```python
from build123d import *

# Parameters (mm, degrees)
SKETCH1_W                = 259.08
SKETCH1_H                = 298.45
BOSS_EXTRUDE3_DEPTH      = 14.732
SKETCH2_W                = 259.08
SKETCH2_H                = 298.45
BOSS_EXTRUDE4_DEPTH      = 22.098
SKETCH4_OUTSIDE_W        = 379.836
SKETCH4_OUTSIDE_H        = 118.216
CUT_EXTRUDE2_DEPTH       = 259.08
SKETCH6_OUTSIDE_W        = 340.466
SKETCH6_OUTSIDE_H        = 118.216
CUT_EXTRUDE4_DEPTH       = 298.45
BOSS_EXTRUDE6_DEPTH      = 101.6
BOSS_EXTRUDE6_DEPTH_BACK = 101.6
SKETCH8_W                = 88.392
SKETCH8_H                = 7.62
CUT_EXTRUDE5_DEPTH       = 127
CUT_EXTRUDE7_DEPTH       = 50.8
CUT_EXTRUDE7_DEPTH_BACK  = 50.8
SKETCH15_W               = 25.4
SKETCH15_H               = 6.576785714
CUT_EXTRUDE8_DEPTH       = 53.086
SKETCH16_W               = 25.4
SKETCH16_H               = 6.576785714
CUT_EXTRUDE9_DEPTH       = 53.086
SKETCH17_R               = 5.08
CUT_EXTRUDE10_DEPTH      = 8.62
SKETCH18_R               = 2.54
CUT_EXTRUDE11_DEPTH      = 260.08
SKETCH19_R               = 5.08
CUT_EXTRUDE12_DEPTH      = 8.62
SKETCH21_R               = 5.08
CUT_EXTRUDE13_DEPTH      = 8.62


with BuildPart() as part:
    # Sketch1 → Boss-Extrude3 (new body)
    with BuildSketch(Plane(origin=(0, 0, 0), x_dir=(1, 0, 0), z_dir=(0, 1, 0))):
        Rectangle(SKETCH1_W, SKETCH1_H)
    extrude(amount=BOSS_EXTRUDE3_DEPTH)

    # Sketch2 → Boss-Extrude4 (add)
    with BuildSketch(Plane.XZ):
        Rectangle(SKETCH2_W, SKETCH2_H)
    extrude(amount=BOSS_EXTRUDE4_DEPTH)

    # Sketch4 outside → Cut-Extrude2 (cut)
    with BuildSketch(Plane(origin=(129.54, 0, 0), x_dir=(0, 0, -1), z_dir=(1, 0, 0))):
        with Locations((0, -3.683)):
            Rectangle(SKETCH4_OUTSIDE_W, SKETCH4_OUTSIDE_H)
        Polygon((0, -22.098), (-149.225, 0), (-149.225, 14.732), (149.225, 14.732), (149.225, 0), align=None, mode=Mode.SUBTRACT)
    extrude(amount=-CUT_EXTRUDE2_DEPTH, mode=Mode.SUBTRACT)

    # Sketch6 outside → Cut-Extrude4 (cut)
    with BuildSketch(Plane.XY.offset(149.225)):
        with Locations((0, -3.683)):
            Rectangle(SKETCH6_OUTSIDE_W, SKETCH6_OUTSIDE_H)
        Polygon((-44.196, -22.098), (44.196, -22.098), (129.54, 0), (129.54, 14.732), (-129.54, 14.732), (-129.54, 0), align=None, mode=Mode.SUBTRACT)
    extrude(amount=-CUT_EXTRUDE4_DEPTH, mode=Mode.SUBTRACT)


with BuildPart() as body_2:
    # Sketch7 → Boss-Extrude6 (new body, two sides)
    with BuildSketch(Plane.XY) as boss_extrude6_sk:
        Polygon((44.196, -27.178), (129.54, -5.08), (129.54, -34.798), (-129.54, -34.798), (-129.54, -5.08), (-44.196, -27.178), align=None)
    extrude(amount=BOSS_EXTRUDE6_DEPTH)
    extrude(boss_extrude6_sk.sketch, amount=-BOSS_EXTRUDE6_DEPTH_BACK)

    # Sketch8 → Cut-Extrude5 (cut)
    with BuildSketch(Plane.XY.offset(101.6)):
        with Locations((0, -30.988)):
            Rectangle(SKETCH8_W, SKETCH8_H)
    extrude(amount=-CUT_EXTRUDE5_DEPTH, mode=Mode.SUBTRACT)

    # Sketch10 → Cut-Extrude7 (cut, two sides)
    with BuildSketch(Plane.XY) as cut_extrude7_sk:
        Polygon((-44.196, -27.178), (-120.396, -7.447642857), (-120.396, -34.798), (-44.196, -34.798), align=None)
        Polygon((120.396, -7.447642857), (44.196, -27.178), (44.196, -34.798), (120.396, -34.798), align=None)
    extrude(amount=CUT_EXTRUDE7_DEPTH, mode=Mode.SUBTRACT)
    extrude(cut_extrude7_sk.sketch, amount=-CUT_EXTRUDE7_DEPTH_BACK, mode=Mode.SUBTRACT)

    # Sketch15 → Cut-Extrude8 (cut)
    with BuildSketch(Plane.XY.offset(101.6)):
        with Locations((56.896, -23.889607143)):
            Rectangle(SKETCH15_W, SKETCH15_H)
    extrude(amount=-CUT_EXTRUDE8_DEPTH, mode=Mode.SUBTRACT)

    # Sketch16 → Cut-Extrude9 (cut)
    with BuildSketch(Plane.XY.offset(101.6)):
        with Locations((-56.896, -23.889607143)):
            Rectangle(SKETCH16_W, SKETCH16_H)
    extrude(amount=-CUT_EXTRUDE9_DEPTH, mode=Mode.SUBTRACT)

    # Sketch17 → Cut-Extrude10 (cut, through all)
    with BuildSketch(Plane(origin=(0, -27.178, 0), x_dir=(1, 0, 0), z_dir=(0, 1, 0))):
        with Locations((-31.496, 88.9)):
            Circle(SKETCH17_R)
        with Locations((31.496, 88.9)):
            Circle(SKETCH17_R)
    extrude(amount=-CUT_EXTRUDE10_DEPTH, mode=Mode.SUBTRACT)

    # Sketch18 → Cut-Extrude11 (cut, through all)
    with BuildSketch(Plane.ZY.offset(129.54)):
        with Locations((38.1, -19.939)):
            Circle(SKETCH18_R)
        with Locations((-38.1, -19.939)):
            Circle(SKETCH18_R)
    extrude(amount=-CUT_EXTRUDE11_DEPTH, mode=Mode.SUBTRACT)

    # Sketch19 → Cut-Extrude12 (cut, through all)
    with BuildSketch(Plane(origin=(0, -27.178, 0), x_dir=(1, 0, 0), z_dir=(0, 1, 0))):
        with Locations((-56.896, -76.2)):
            Circle(SKETCH19_R)
    extrude(amount=-CUT_EXTRUDE12_DEPTH, mode=Mode.SUBTRACT)

    # Sketch21 → Cut-Extrude13 (cut, through all)
    with BuildSketch(Plane(origin=(0, -27.178, 0), x_dir=(1, 0, 0), z_dir=(0, 1, 0))):
        with Locations((56.896, -76.2)):
            Circle(SKETCH21_R)
    extrude(amount=-CUT_EXTRUDE13_DEPTH, mode=Mode.SUBTRACT)


solid = body_2.part
```
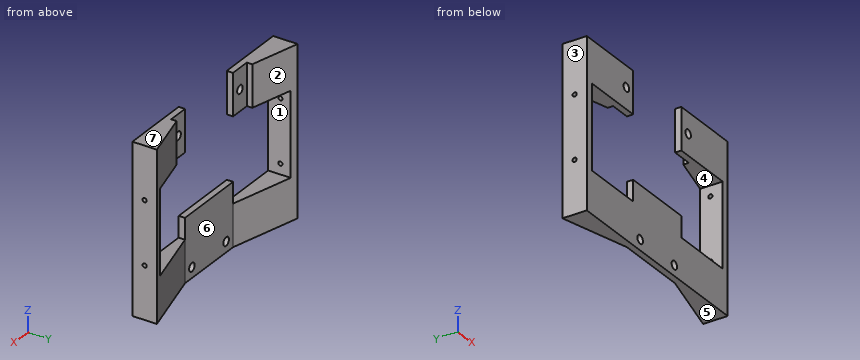
Part model, mm, in its own coordinate system. Face numbers are marked on the shaded views. A direction names the side the tool comes from. Round coordinates to 2 decimals unless told otherwise and drop trailing zeros. Loops run counter-clockwise (first coordinate to the right, second up) from the corner with the lowest first, then second, coordinate; pieces in that order, holes last.
Item 1: Mould opens along Z. For the marked faces 4, 5, 6 and 7 say: +Z half, -Z half, draft (parallel to the pull), parting line (faces both ways), or undercut.
Item 2: Cut at C-C, the plane x = 88. Give the cut face in (y, z), then the cut area to 3 significant figures.
Item 3: Drill centre lines: line 1 (X direction, y = -31.5, z = -88.9); line 2 (X direction, y = -14.25, z = -19.5); line 3 (X direction, y = -30, z = 76.2). Where is each one in solid material? Low to high.
Item 4: Cut at B-B, the plane z = 76.2. Give the cut face in (x, y), then the cut area to 3 significant figures.
Item 5: Cut at A-A, the plane z = -88.9. Give the cut face in (x, y).
Item 6: Drop flat-ended pins along their axis: P1, Ø20.5, axis at x = -56, z = 70, coming from the +Y side; P2, Ø6, axis at x = 17.5, y = -30, coming from the +Z side. Give the stop position or say it passes through.
Item 7: 3-axis set-ups, long thin cutter, end or side, ignore diameter. For the marked faces 1, 2 and 3: which of +Z, -Z, +X, -X, +Y, -Y reach the whole face in a straight line?
Item 8: Cut at D-D, the plane x = 54.5. Give the cut face in (y, z).
A:
1. face 4: undercut
1. face 5: -Z half
1. face 6: draft
1. face 7: +Z half
2. outline: (-34.8, -101.6) - (-15.84, -101.6) - (-15.84, -50.8) - (-34.8, -50.8) - close; (-34.8, 50.8) - (-15.84, 50.8) - (-15.84, 101.6) - (-34.8, 101.6) - close
2. area: 1,930 mm2
3. line 1: x = -129.54 to -36.58, -26.42 to 26.42, 36.58 to 129.54
3. line 2: x = -129.54 to -120.4, 120.4 to 129.54
3. line 3: x = -129.54 to -61.98, -51.82 to -44.2, 44.2 to 51.82, 61.98 to 129.54
4. outline: (-129.54, -34.8) - (-61.98, -34.8) - (-61.98, -27.18) - (-69.6, -27.18) - (-69.6, -20.6) - (-129.54, -5.08) - close; (-51.82, -34.8) - (-44.2, -34.8) - (-44.2, -27.18) - (-51.82, -27.18) - close; (44.2, -34.8) - (51.82, -34.8) - (51.82, -27.18) - (44.2, -27.18) - close; (61.98, -34.8) - (129.54, -34.8) - (129.54, -5.08) - (69.6, -20.6) - (69.6, -27.18) - (61.98, -27.18) - close
4. area: 2,860 mm2
5. outline: (-129.54, -34.8) - (-36.58, -34.8) - (-36.58, -27.18) - (-44.2, -27.18) - (-129.54, -5.08) - close; (-26.42, -34.8) - (26.42, -34.8) - (26.42, -27.18) - (-26.42, -27.18) - close; (36.58, -34.8) - (129.54, -34.8) - (129.54, -5.08) - (44.2, -27.18) - (36.58, -27.18) - close
6. P1: stops at y = -27.18
6. P2: stops at z = -25.4
7. face 1: +Y, -Y
7. face 2: +Z, -Z, +Y
7. face 3: +Z, -Z, -X, +Y, -Y
8. outline: (-34.8, -101.6) - (-24.51, -101.6) - (-24.51, -50.8) - (-34.8, -50.8) - close; (-34.8, 50.8) - (-27.18, 50.8) - (-27.18, 71.72) - (-34.8, 71.72) - close; (-34.8, 80.68) - (-27.18, 80.68) - (-27.18, 101.6) - (-34.8, 101.6) - close
